Read the model definition and answer for the solid it produces. Units are mm, in the model's axes. A direction names the side the tool comes from. Give positions to 0.01 mm unless a question says otherwise; leave off trailing zeros. Write each loop counter-clockwise with the first axis right and the second up, starting at its lowest first coordinate (ties: lowest second). Pieces come first, ordered by that corner, then holes. Notation, with made-up numbers: (34, 12.5) -> (61, 12.5) arc R21 ccw to (61, 42.5) -> close; hole circle Ø5 at (25.5, -35.75). An arc over 180 degrees is marked (long way). Put each result on its own line as item: value. Start each with the question number.
from build123d import *

# Parameters (mm, degrees)
F0_W     = 140
F0_H     = 40
F0_R     = 8
F1_DEPTH = 5
F2_W     = 140
F2_H     = 5
F3_DEPTH = 55
F4_W     = 5
F4_H     = 30
F5_DEPTH = 55
F6_R     = 2.5
F7_DEPTH = 60


with BuildPart() as f1:
    # F0 (on Top) → F1 (new body)
    with BuildSketch(Plane.XY):
        Rectangle(F0_W, F0_H)
        with Locations((-45, -4)):
            Circle(F0_R, mode=Mode.SUBTRACT)
        with Locations((0, -4)):
            Circle(F0_R, mode=Mode.SUBTRACT)
        with Locations((45, -4)):
            Circle(F0_R, mode=Mode.SUBTRACT)
    extrude(amount=F1_DEPTH)

    # F2 (on face) → F3 (join)
    with BuildSketch(Plane(origin=(0, 0, 0), x_dir=(1, 0, 0), z_dir=(0, 0, -1))):
        with Locations((0, 17.5)):
            Rectangle(F2_W, F2_H)
        with Locations((0, -17.5)):
            Rectangle(F2_W, F2_H)
    extrude(amount=F3_DEPTH)

    # F4 (on face) → F5 (join)
    with BuildSketch(Plane(origin=(0, 0, 0), x_dir=(1, 0, 0), z_dir=(0, 0, -1))):
        with Locations((-67.5, 0)):
            Rectangle(F4_W, F4_H)
        with Locations((67.5, 0)):
            Rectangle(F4_W, F4_H)
    extrude(amount=F5_DEPTH)

    # F6 (on face) → F7 (cut)
    with BuildSketch(Plane.XZ.offset(20)):
        with Locations((10, -50)):
            Circle(F6_R)
        with Locations((-10, -50)):
            Circle(F6_R)
    extrude(amount=-F7_DEPTH, mode=Mode.SUBTRACT)


solid = f1.part
1) For faces 1 (the face through (-1, -15, -27)), 2 (the face through (9.46, -17.54, -52.44)), determine the directions among +Z, -Z, +X, -X, +Y, -Y from which every point of the face is accessible in a straight line to the end or side of a thin tool.
2) A cutting plane is placed at D-D on z = -50. Give the vertices of the cut face in (x, y), and give its area (3 significant figures).
3) Straight lines are drawn through the part: line 1 (X direction, y = -11, z = -50.5); line 2 (Z direction, x = -10, y = -18); line 3 (Y direction, x = -49, z = -6). For each, find the intervals that lie inside material, in ascending order. Write a range as [from, to].
4) A cutting plane is placed at A-A on x = 10. Give the vertices of the cut face in (y, z), and give its area (3 significant figures).
5) Each of these flat-tipped pins is pushed along its axis until it touches: pin 1 Ø4.5 at (x, z) = (10, -50) entering from +Y; pin 2 Ø21 at (x, y) = (0, -4) entering from -Z. Where does it stop, or does it pass through?
6) A cutting plane is placed at B-B on y = -4. Give the vertices of the cut face in (x, z), and give its area (3 significant figures).
7) For a pull along Z with two mould halves and no side action, classify faces 3 (the face through (9.46, 17.47, -52.44)), 4 (the face through (65, 0, -27)), 5 (the face through (-6, 16, -55)) as pulls with the +Z half, pulls with the -Z half, needs draft (parallel to the pull), parting line crosses it, or undercut.
8) A cutting plane is placed at C-C on z = -43.5. Give the vertices of the cut face in (x, y).
Results found:
1. face 1: -Z
1. face 2: +Y, -Y
2. outline: (-70, -20) -> (-12.5, -20) -> (-12.5, -15) -> (-65, -15) -> (-65, 15) -> (-12.5, 15) -> (-12.5, 20) -> (-70, 20) -> close; (-7.5, -20) -> (7.5, -20) -> (7.5, -15) -> (-7.5, -15) -> close; (-7.5, 15) -> (7.5, 15) -> (7.5, 20) -> (-7.5, 20) -> close; (12.5, -20) -> (70, -20) -> (70, 20) -> (12.5, 20) -> (12.5, 15) -> (65, 15) -> (65, -15) -> (12.5, -15) -> close
2. area: 1,600 mm²
3. line 1: x = [-70, -65], [65, 70]
3. line 2: z = [-55, -52.5], [-47.5, 5]
3. line 3: y = [-20, -15], [15, 20]
4. outline: (-20, -55) -> (-15, -55) -> (-15, -52.5) -> (-20, -52.5) -> close; (-20, -47.5) -> (-15, -47.5) -> (-15, 0) -> (15, 0) -> (15, -47.5) -> (20, -47.5) -> (20, 5) -> (-20, 5) -> close; (15, -55) -> (20, -55) -> (20, -52.5) -> (15, -52.5) -> close
4. area: 700 mm²
5. pin 1: passes through
5. pin 2: stops at z = 0
6. outline: (-70, -55) -> (-65, -55) -> (-65, 0) -> (-53, 0) -> (-53, 5) -> (-70, 5) -> close; (-37, 0) -> (-8, 0) -> (-8, 5) -> (-37, 5) -> close; (8, 0) -> (37, 0) -> (37, 5) -> (8, 5) -> close; (53, 0) -> (65, 0) -> (65, -55) -> (70, -55) -> (70, 5) -> (53, 5) -> close
6. area: 1,010 mm²
7. face 3: undercut
7. face 4: needs draft
7. face 5: pulls with the -Z half
8. outline: (-70, -20) -> (70, -20) -> (70, 20) -> (-70, 20) -> close; hole (-65, -15) -> (65, -15) -> (65, 15) -> (-65, 15) -> close
